Model file for the job. Use its own axes, mm. Face numbers are marked on the shaded views. Coordinates: 2 decimals unless noted, no trailing zeros. Order: outer loops, then holes, each group sorted by start corner. A loop starts at its lowest first (then second) coordinate and runs counter-clockwise, first axis right, second up. Notation, with made-up numbers: (5, 70) -> (20, 70) arc R7 cw to (20, 79) -> close; hole circle Ø10 at (23.25, 68.25). An arc over 180 degrees is marked (long way). Write item = value, one per line. Start each with the question number.
Q1. Cut at B-B, the plane y = -38.5. List the corners of the cut face in (x, z).
Q2. Cut at C-C, the plane z = 0.8. Give the number of separate pieces and of enclosed holes in the cut face, plus the area to 3 significant figures.
Q3. Wall check: line 1 (Y direction, x = -40, z = 1.05); line 2 (Y direction, x = -22.5, z = 2.15); line 3 (Y direction, x = -23.5, z = 0.6). Give the ranges that are in metal, low to high. Write a range as from..to.
Q4. Cut at D-D, the plane y = -75. List the corners of the cut face in (x, z).
Q5. Mould opens along Y. For the marked faces 1 and 2 say: +Y half, -Y half, draft (parallel to the pull), parting line (faces both ways), or undercut.
Q6. Cut at A-A, the plane y = 0. List the corners of the cut face in (x, z).
Q7. Flat gauge pins, fed straight in: pin 1 (5 mm diameter, centred on x = -40, y = 85, fed in from -Z); pin 2 (10.5 mm diameter, centred on x = -13, y = -59, fed in from +Z); pin 3 (0.9 mm diameter, centred on x = -1.5, z = 1, fed in from +Y); pin 4 (1.5 mm diameter, centred on y = -13, z = 1.5, fed in from -X). Where does each tip first touch, or does it go through?
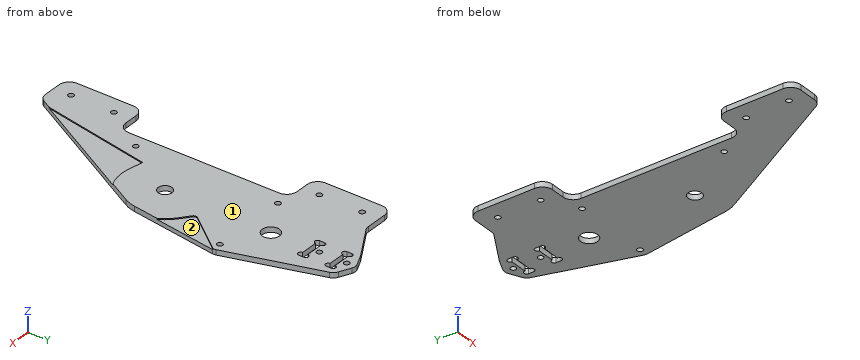
Autodesk Inventor part; units mm, degrees
ref_plane "YZ Plane" through (0, 0, 0) normal (1, 0, 0) x (0, 1, 0)
ref_plane "XZ Plane" through (0, 0, 0) normal (0, 1, 0) x (-1, 0, 0)
ref_plane "XY Plane" through (0, 0, 0) normal (0, 0, 1) x (1, 0, 0)
sketch "スケッチ1" plane through (0, 0, 0) normal (0, 0, 1) x (1, 0, 0)
  arc A0 (0, -120) -> (0, 120) centre (0, 0) ccw
  line L0 (0, 120) -> (0, -120)
  dimension "d0" = 120
extrude "押し出し1" add sketch "スケッチ1" along normal blind 3
sketch "スケッチ2" plane through (0, 0, 0) normal (0, 0, -1) x (-1, 0, 0)
  line L0 (0, 120) -> (0, -120)
  line L1 (0, 120) -> (50, 120)
  line L2 (50, 120) -> (50, -120)
  line L3 (50, -120) -> (0, -120)
  line L4 (0, -120) -> (0, 120)
  point P0 (0, 0)
  dimension "d3" = 50
extrude "押し出し2" add sketch "スケッチ2" against normal blind 3
sketch "スケッチ3" plane through (0, 0, 3) normal (0, 0, 1) x (1, 0, 0)
  line L0 (-50, 120) -> (-50, -120)
  line L1 (-50, 40) -> (-40, 40)
  line L2 (-40, 40) -> (-40, -40)
  line L3 (-40, -40) -> (-50, -40)
  line L4 (-50, -40) -> (-50, 40)
  line L5 (-40, 60) -> (-40, -60) construction
  circle A0 centre (-40, 60) radius 1.6
  circle A1 centre (-40, -60) radius 1.6
  point P0 (0, 0)
  point P1 (-50, 0)
  point P2 (-40, 0)
  point P3 (-40, 0)
  dimension "d8" = 10
  dimension "d9" = 80
  dimension "d10" = 120
  dimension "d11" = 10
  dimension "d12" = 3.2
  dimension "d13" = 3.2
extrude "押し出し3" cut sketch "スケッチ3" against normal through all
sketch "スケッチ4" plane through (0, 0, 3) normal (0, 0, 1) x (1, 0, 0)
  circle A0 centre (0, 0) radius 4
  dimension "d14" = 8
extrude "押し出し4" cut sketch "スケッチ4" against normal blind 3
sketch "スケッチ5" plane through (0, 0, 3) normal (0, 0, 1) x (1, 0, 0)
  circle A0 centre (0, 61.8122) radius 3
  circle A1 centre (0, 61.8122) radius 5
  point P0 (0, 0)
  dimension "d17" = 10
extrude "押し出し5" cut sketch "スケッチ5" against normal blind 3 contours A0 | A1
sketch "スケッチ7" plane through (0, 0, 3) normal (0, 0, 1) x (1, 0, 0)
  line L0 (15.7, 89.1122) -> (-15.7, 89.1122)
  line L1 (8, 87.1122) -> (-8, 87.1122)
  line L2 (-8, 87.1122) -> (-8, 84.1122)
  line L3 (-8, 84.1122) -> (8, 84.1122)
  line L4 (8, 84.1122) -> (8, 87.1122)
  arc A0 (-8, 84.1122) -> (-5, 84.1122) centre (-6.5, 84.1122) ccw
  arc A1 (5, 84.1122) -> (8, 84.1122) centre (6.5, 84.1122) ccw
  arc A2 (8, 87.1122) -> (5, 87.1122) centre (6.5, 87.1122) ccw
  arc A3 (-5, 87.1122) -> (-8, 87.1122) centre (-6.5, 87.1122) ccw
  circle A4 centre (0, 90.1122) radius 1.6
  point P0 (0, 0)
  point P1 (0, 87.1122)
  point P2 (0, 89.1122)
  dimension "d20" = 2
  dimension "d21" = 16
  dimension "d22" = 3
  dimension "d23" = 1.5
  dimension "d26" = 3.2
  dimension "d27" = 3
extrude "押し出し6" cut sketch "スケッチ7" against normal blind 3
pattern_linear "矩形状パターン1" count 2 spacing 16 along (0, 1, 0) of "押し出し6"
sketch "スケッチ9" plane through (0, 0, 3) normal (0, 0, 1) x (1, 0, 0)
  circle A0 centre (0, 61.8122) radius 4 construction
  circle A1 centre (0, 0) radius 4 construction
  circle A2 centre (22.5, 49) radius 1.6
  circle A3 centre (-22.5, -34) radius 1.6
  circle A4 centre (-22.5, 49) radius 1.6
  line L0 (25.0237, 50.6221) -> (12.6183, 69.9225) construction
  arc A5 (12.6183, 69.9225) -> (-12.6183, 69.9226) centre (0, 61.8122) ccw construction
  line L1 (-12.6183, 69.9226) -> (-25.0237, 50.6221) construction
  arc A6 (-25.0237, 50.6221) -> (-25.5, 49) centre (-22.5, 49) ccw construction
  line L2 (-25.5, 49) -> (-25.5, -34) construction
  arc A7 (-25.5, -34) -> (-20.5963, -36.3186) centre (-22.5, -34) ccw construction
  line L3 (-20.5963, -36.3186) -> (9.5184, -11.5931) construction
  arc A8 (9.5184, -11.5931) -> (14.6828, -3.0686) centre (0, 0) ccw construction
  line L4 (14.6828, -3.0686) -> (25.4366, 48.3863) construction
  arc A9 (25.4366, 48.3863) -> (25.0237, 50.6221) centre (22.5, 49) ccw construction
  point P0 (0, 0)
extrude "押し出し8" cut sketch "スケッチ9" against normal blind 3
sketch "スケッチ8" plane through (0, 0, 3) normal (0, 0, 1) x (1, 0, 0)
  arc A0 (17.4743, -9.7287) -> (19.7797, -2.9601) centre (0, 0) ccw
  line L0 (17.4743, -9.7287) -> (-30, -95)
  circle A1 centre (22.5, 49) radius 1.6
  circle A2 centre (-22.5, 49) radius 1.6
  circle A3 centre (-22.5, -34) radius 1.6
  arc A4 (27.4449, 48.26) -> (27.2948, 50.4177) centre (22.5, 49) ccw
  line L1 (27.4449, 48.26) -> (19.7797, -2.9601)
  arc A5 (11.2948, 104.5299) -> (8.5953, 107.652) centre (6.5, 103.1122) ccw
  arc A6 (2.0953, 110.652) -> (-2.0953, 110.652) centre (0, 106.1122) ccw
  line L2 (8.5953, 107.652) -> (2.0953, 110.652)
  line L3 (27.2948, 50.4177) -> (11.2948, 104.5299)
  line L4 (-2.0953, 110.652) -> (-8.5953, 107.652)
  arc A7 (-8.5953, 107.652) -> (-9.0487, 107.4138) centre (-6.5, 103.1122) ccw
  line L5 (-9.0487, 107.4138) -> (-30, 95)
  circle A8 centre (-40, 85) radius 1.6
  line L6 (-50, 50) -> (-30, 50)
  line L7 (-30, 95) -> (-30, 50)
  line L8 (-50, 95) -> (-30, 95)
  line L9 (-50, 50) -> (-50, 95)
  circle A9 centre (-40, 60) radius 1.6
  circle A10 centre (-40, -85) radius 1.6
  circle A11 centre (-40, -60) radius 1.6
  line L10 (-30, -50) -> (-50, -50)
  line L11 (-50, -95) -> (-50, -50)
  line L12 (-30, -95) -> (-50, -95)
  line L13 (-30, -50) -> (-30, -95)
  line L14 (-30, 50) -> (-30, -50)
  point P0 (-47, -55)
  point P1 (-50, -80)
  point P2 (-35, 50)
  point P3 (-35, 95)
  point P4 (-35, -50)
  point P5 (-35, -95)
  dimension "d41" = 10
  dimension "d44" = 5
  dimension "d48" = 20
extrude "押し出し9" cut sketch "スケッチ8" against normal through all contours L0 L13 L14 L7 L5 A7 L4 A6 L2 A5 L3 A4 L1 A0 | L12 L11 L10 L13 | L6 L9 L8 L7 | A1 | A2 | A3 keep common part
fillet "フィレット2" radius 6 8 edges at (-50, 50, 1.5) (-30, 50, 1.5) (-30, -50, 1.5) (-50, -50, 1.5) (-50, 95, 1.5) (-30, 95, 1.5) (-50, -95, 1.5) (-30, -95, 1.5)
sketch "スケッチ10" plane through (0, 0, 3) normal (0, 0, 1) x (1, 0, 0)
  arc A0 (-33.5268, -95) -> (-28.2845, -91.9186) centre (-33.5268, -89) ccw
  line L0 (17.4743, -9.7287) -> (-28.2845, -91.9186)
  arc A1 (17.4743, -9.7287) -> (19.7797, -2.9601) centre (0, 0) ccw
  line L1 (27.4449, 48.26) -> (19.7797, -2.9601)
  arc A2 (27.4449, 48.26) -> (27.2948, 50.4177) centre (22.5, 49) ccw
  line L2 (11.2948, 104.5299) -> (27.2948, 50.4177)
  arc A3 (11.2948, 104.5299) -> (8.5953, 107.652) centre (6.5, 103.1122) ccw
  line L3 (2.0953, 110.652) -> (8.5953, 107.652)
  arc A4 (2.0953, 110.652) -> (-2.0953, 110.652) centre (0, 106.1122) ccw
  line L4 (-8.5953, 107.652) -> (-2.0953, 110.652)
  arc A5 (-8.5953, 107.652) -> (-9.0487, 107.4138) centre (-6.5, 103.1122) ccw
  line L5 (-28.5856, 95.8381) -> (-9.0487, 107.4138)
  arc A6 (-31.6441, 95) -> (-28.5856, 95.8381) centre (-31.6441, 101) ccw
  line L6 (-44, 95) -> (-31.6441, 95)
  arc A7 (-44, 95) -> (-50, 89) centre (-44, 89) ccw
  line L7 (-50, 89) -> (-50, 56)
  arc A8 (-50, 56) -> (-44, 50) centre (-44, 56) ccw
  line L8 (-36, 50) -> (-44, 50)
  arc A9 (-30, 44) -> (-36, 50) centre (-36, 44) ccw
  line L9 (-30, -44) -> (-30, 44)
  arc A10 (-36, -50) -> (-30, -44) centre (-36, -44) ccw
  line L10 (-44, -50) -> (-36, -50)
  arc A11 (-44, -50) -> (-50, -56) centre (-44, -56) ccw
  line L11 (-50, -56) -> (-50, -89)
  arc A12 (-50, -89) -> (-44, -95) centre (-44, -89) ccw
  line L12 (-33.5268, -95) -> (-44, -95)
  circle A13 centre (-40, -85) radius 1.6
  circle A14 centre (-40, 85) radius 1.6
  circle A15 centre (-22.5, -34) radius 1.6
  circle A16 centre (22.5, 49) radius 1.6
  circle A17 centre (-22.5, 49) radius 1.6
  circle A18 centre (0, 106.1122) radius 1.6
  arc A19 (8, 103.1122) -> (5, 103.1122) centre (6.5, 103.1122) ccw
  line L13 (8, 103.1122) -> (8, 100.1122)
  arc A20 (5, 100.1122) -> (8, 100.1122) centre (6.5, 100.1122) ccw
  line L14 (5, 100.1122) -> (-5, 100.1122)
  arc A21 (-8, 100.1122) -> (-5, 100.1122) centre (-6.5, 100.1122) ccw
  line L15 (-8, 100.1122) -> (-8, 103.1122)
  arc A22 (-5, 103.1122) -> (-8, 103.1122) centre (-6.5, 103.1122) ccw
  line L16 (-5, 103.1122) -> (5, 103.1122)
  circle A23 centre (0, 90.1122) radius 1.6
  arc A24 (8, 87.1122) -> (5, 87.1122) centre (6.5, 87.1122) ccw
  line L17 (8, 87.1122) -> (8, 84.1122)
  arc A25 (5, 84.1122) -> (8, 84.1122) centre (6.5, 84.1122) ccw
  line L18 (5, 84.1122) -> (-5, 84.1122)
  arc A26 (-8, 84.1122) -> (-5, 84.1122) centre (-6.5, 84.1122) ccw
  line L19 (-8, 84.1122) -> (-8, 87.1122)
  arc A27 (-5, 87.1122) -> (-8, 87.1122) centre (-6.5, 87.1122) ccw
  line L20 (-5, 87.1122) -> (5, 87.1122)
  circle A28 centre (0, 61.8122) radius 5
  circle A29 centre (0, 0) radius 4
  circle A30 centre (-40, 60) radius 1.6
  circle A31 centre (-40, -60) radius 1.6
  line L21 (27.4974, 48.8393) -> (9.9725, 26.4915)
  circle A32 centre (66.9129, -143.1316) radius 1.6
  circle A33 centre (14.399, -30.8005) radius 1.6
  circle A34 centre (20.7515, -44.3889) radius 1.6
  circle A35 centre (58.443, -125.0137) radius 1.6
  line L22 (4.2168, -26.7296) -> (17.8052, -20.3771)
  line L23 (4.2168, -26.7296) -> (63.5067, -153.555)
  line L24 (77.0952, -147.2025) -> (63.5067, -153.555)
  line L25 (17.8052, -20.3771) -> (77.0952, -147.2025)
  line L26 (15.427, 19.6725) -> (10.3121, 23.6835)
  arc A36 (9.9725, 26.4915) -> (10.3121, 23.6835) centre (11.5463, 25.2573) ccw
  circle A37 centre (-26.1999, -135.4901) radius 1.6
  circle A38 centre (-6.455, -33.3816) radius 1.6
  circle A39 centre (-9.3028, -48.1088) radius 1.6
  circle A40 centre (-23.352, -120.7629) radius 1.6
  line L27 (-12.2998, -24.1032) -> (2.4274, -26.951)
  line L28 (-12.2998, -24.1032) -> (-35.0823, -141.9207)
  line L29 (-20.3551, -144.7685) -> (-35.0823, -141.9207)
  line L30 (2.4274, -26.951) -> (-20.3551, -144.7685)
  line L31 (-4.7464, -24.5453) -> (-13.0918, -22.9315)
  line L32 (-13.0918, -22.9315) -> (-25.446, -86.8203)
  arc A41 (-4.7464, -24.5453) -> (10.1778, -22.8345) centre (0, 0) ccw
  arc A42 (21.9998, 11.8747) -> (15.427, 19.6725) centre (0, 0) ccw
  dimension "d54" = 2
  dimension "d55" = 1
  dimension "d56" = 1
  dimension "d57" = 25
extrude "押し出し11" cut sketch "スケッチ10" against normal blind 0.6 contours L32 L31 A41 L0 L22 L23 L30 L27 L28 | L28 L27 L30 L0 | L23 L22 L0 | A42 L26 A36 L21 A2 L1 | A33 | A38 | A39
properties part number "Pitch_B" material "アルミニウム"
Here are the results:
q1.outline = (-30, 0) -> (1.46, 0) -> (1.46, 2.4) -> (-16.1, 2.4) -> (-16.1, 3) -> (-30, 3) -> close
q2.separate_pieces = 1
q2.enclosed_holes = 13
q2.area = 9,370 mm²
q3.line_1 = -95..-86.6, -83.4..-61.6, -58.4..-50, 50..58.4, 61.6..83.4, 86.6..95
q3.line_2 = -81.53..-35.6, -32.4..47.4, 50.6..99.44
q3.line_3 = -83.32..-35.25, -32.75..47.75, 50.25..98.85
q4.outline = (-50, 0) -> (-18.87, 0) -> (-18.87, 2.4) -> (-23.16, 2.4) -> (-23.16, 3) -> (-50, 3) -> close
q5.face_1 = draft
q5.face_2 = undercut
q6.outline = (-30, 0) -> (-4, 0) -> (-4, 3) -> (-30, 3) -> close; (4, 0) -> (20.22, 0) -> (20.22, 3) -> (4, 3) -> close
q7.pin_1 = 0
q7.pin_2 = 2.4
q7.pin_3 = 111
q7.pin_4 = -30
